Here's how the part is built. I have some questions about the finished solid (model axes, mm). A direction names the side the tool comes from. Give positions to 0.01 mm unless a question says otherwise; leave off trailing zeros. Write each loop counter-clockwise with the first axis right and the second up, starting at its lowest first coordinate (ties: lowest second). Pieces come first, ordered by that corner, then holes. Notation, with made-up numbers: M 25,32.5 L 59,32.5 A14 ccw 59,53.5 Z; hole C -26,56.5 d8. An arc over 180 degrees is marked long. Answer as CSV lines item,"result". Start each with the question number.
Q1. Suppose I cut it at B-B (z = 4). Write out the boundary of the cut face in (x, y), then the cut area to 3 significant figures.
Q2. On a 3-axis mill with a long thin cutter (end or side, diameter ignored), from which of +Z, -Z, +X, -X, +Y, -Y can I reach the whole of each face in a straight line? I mean faces 1 (the cylindrical face through (147.689, 9.598, -62.764)), 2 (the flat face through (148, 2, -87)), 3 (the flat face through (15, 2, -30)). Say none if no direction works.
Q3. Suppose I cut it at C-C (x = 89.25). Write out the boundary of the cut face in (y, z), then the cut area to 3 significant figures.
Q4. Thinking about a two-plate mould opening in X: for faces 4 (the flat face through (36, 2, 0)), 5 (the flat face through (20, 2, -66)), 6 (the flat face through (15, 2, -62)), 7 (the flat face through (37, 2, -67)), which applies, +X half, -X half, draft (parallel to the pull), parting line (faces both ways), or undercut?
Q5. For pin 1 (3.5 mm diameter, centred on x = 27.5, y = 1, fed in from -Z); pin 2 (2 mm diameter, centred on x = 155, y = 1.5, fed in from -Z); pin 3 (1 mm diameter, centred on y = 12, z = -26, fed in from -X), each with a flat end and sliding along its axis, tell me the tip position at first contact or that it passes through.
Q6. Suppose I cut it at A-A (x = 49.5). Write out the boundary of the cut face in (y, z), then the cut area to 4 significant figures.
Q7. If I drill on line 1 along Z through (x, y) = (145.75, 10.25); line 2 along X through (y, z) = (9, 4); line 3 along Z through (x, y) = (145, 1), over which ranges is the centre line in solid material (lowest first)?
```python
from build123d import *
from OCP.BRepFilletAPI import BRepFilletAPI_MakeChamfer

# Parameters (mm, degrees)
SKETCH1_W                       = 180
SKETCH1_H                       = 60
SKETCH1_W_2                     = 150
SKETCH1_H_2                     = 35
BOSS_EXTRUDE1_DEPTH             = 4.5
FILLET1_R                       = 5
FILLET2_R                       = 2
BOSS_EXTRUDE2_DEPTH             = 4.5
CHAMFER1_SIZE                   = 25
CHAMFER2_SIZE                   = 2
BOSS_EXTRUDE3_DEPTH             = 12
BOSS_EXTRUDE3_DIRECTION_2_REACH = 205.581
CHAMFER3_SIZE                   = 10
CHAMFER3_SIZE_2                 = 12
CHAMFER4_SIZE                   = 8
BOSS_EXTRUDE4_START             = 8
BOSS_EXTRUDE4_DEPTH             = 8
SKETCH5_R                       = 2.3
CUT_EXTRUDE1_DEPTH              = 14
CHAMFER5_SIZE                   = 12
CHAMFER5_SIZE2                  = 10
SKETCH6_W                       = 20
SKETCH6_H                       = 10
SKETCH6_W_2                     = 14
SKETCH6_H_2                     = 6
BOSS_EXTRUDE5_DEPTH             = 4.5
CHAMFER6_SIZE                   = 4
SKETCH7_W                       = 14
SKETCH7_H                       = 2.25
CUT_EXTRUDE2_DEPTH              = 3


with BuildPart() as part:
    # Sketch1 → Boss-Extrude1 (new body)
    with BuildSketch(Plane(origin=(0, 0, 0), x_dir=(1, 0, 0), z_dir=(0, 1, 0))):
        with Locations((90, 30)):
            Rectangle(SKETCH1_W, SKETCH1_H)
        with Locations((90, 30)):
            Rectangle(SKETCH1_W_2, SKETCH1_H_2, mode=Mode.SUBTRACT)
    extrude(amount=BOSS_EXTRUDE1_DEPTH)

    # Fillet1
    fillet1_edges = [part.edges().sort_by_distance(p)[0] for p in [
        (0, 2.25, -60),
        (180, 2.25, 0),
        (0, 2.25, 0),
    ]]
    fillet(fillet1_edges, radius=FILLET1_R)

    # Fillet2
    fillet2_edges = [part.edges().sort_by_distance(p)[0] for p in [
        (165, 2.25, -12.5),
        (165, 2.25, -47.5),
        (15, 2.25, -47.5),
        (15, 2.25, -12.5),
    ]]
    fillet(fillet2_edges, radius=FILLET2_R)

    # Sketch2 → Boss-Extrude2 (add)
    with BuildSketch(Plane(origin=(0, 4.5, 0), x_dir=(1, 0, 0), z_dir=(0, 1, 0))):
        Polygon((180, 80), (180, 60), (136, 60), (136, 80), (136, 95), (148, 95), (148, 80), (168, 80), (168, 95), (180, 95), align=None)
    extrude(amount=-BOSS_EXTRUDE2_DEPTH)

    # Chamfer1
    chamfer1_edges = [part.edges().sort_by_distance(p)[0] for p in [
        (136, 2.25, -60),
    ]]
    chamfer(chamfer1_edges, length=CHAMFER1_SIZE)

    # Chamfer2
    chamfer2_edges = [part.edges().sort_by_distance(p)[0] for p in [
        (168, 2.25, -95),
        (148, 2.25, -95),
    ]]
    chamfer(chamfer2_edges, length=CHAMFER2_SIZE)

    # Sketch3 → Boss-Extrude3 (add)
    with BuildSketch(Plane(origin=(0, 4.5, 0), x_dir=(1, 0, 0), z_dir=(0, 1, 0))):
        Polygon((90, -8), (160, -8), (160, 0), (90, 0), (75, 0), (75, -8), align=None)
        Polygon((160, 60), (90, 60), (75, 60), (75, 68), (90, 68), (160, 68), align=None)
    extrude(amount=BOSS_EXTRUDE3_DEPTH)

    # Boss-Extrude3 direction 2: up to this face of the body (flat: up to its plane)
    boss_extrude3_direction_2_end = Plane(part.part.faces().sort_by_distance((141, 0, -92.964686756))[0])
    # Sketch3 → Boss-Extrude3 direction 2 (add, up to the picked face)
    with BuildSketch(Plane(origin=(0, 4.5, 0), x_dir=(1, 0, 0), z_dir=(0, 1, 0)), mode=Mode.PRIVATE) as boss_extrude3_direction_2_sk1:
        Polygon((90, -8), (160, -8), (160, 0), (90, 0), (75, 0), (75, -8), align=None)
    boss_extrude3_direction_2_tool1 = split(extrude(boss_extrude3_direction_2_sk1.sketch, amount=-BOSS_EXTRUDE3_DIRECTION_2_REACH, mode=Mode.PRIVATE), bisect_by=boss_extrude3_direction_2_end, keep=Keep.BOTH, mode=Mode.PRIVATE)
    # Sketch3 → Boss-Extrude3 direction 2 (add, up to the picked face)
    with BuildSketch(Plane(origin=(0, 4.5, 0), x_dir=(1, 0, 0), z_dir=(0, 1, 0)), mode=Mode.PRIVATE) as boss_extrude3_direction_2_sk2:
        Polygon((160, 60), (90, 60), (75, 60), (75, 68), (90, 68), (160, 68), align=None)
    boss_extrude3_direction_2_tool2 = split(extrude(boss_extrude3_direction_2_sk2.sketch, amount=-BOSS_EXTRUDE3_DIRECTION_2_REACH, mode=Mode.PRIVATE), bisect_by=boss_extrude3_direction_2_end, keep=Keep.BOTH, mode=Mode.PRIVATE)
    add(boss_extrude3_direction_2_tool1.solids().sort_by(Axis((117.5, 4.5, 4), (0, -1, 0)))[0])
    add(boss_extrude3_direction_2_tool2.solids().sort_by(Axis((117.5, 4.5, -64), (0, -1, 0)))[0])

    # Chamfer3
    chamfer3_edges_1 = [part.edges().sort_by_distance(p)[0] for p in [
        (160, 16.5, -64),
    ]]
    chamfer3_side_1 = [part.faces().sort_by_distance(p)[0] for p in [
        (159.8, 16.5, -64),
    ]]
    chamfer3_edges_2 = [part.edges().sort_by_distance(p)[0] for p in [
        (75, 16.5, -64),
    ]]
    chamfer3_side_2 = [part.faces().sort_by_distance(p)[0] for p in [
        (75.2, 16.5, -64),
    ]]
    chamfer3_edges_3 = [part.edges().sort_by_distance(p)[0] for p in [
        (75, 16.5, 4),
    ]]
    chamfer3_side_3 = [part.faces().sort_by_distance(p)[0] for p in [
        (75.2, 16.5, 4),
    ]]
    chamfer3 = BRepFilletAPI_MakeChamfer(part.part.solid().wrapped)
    for e in chamfer3_edges_1:
        chamfer3.Add(CHAMFER3_SIZE - 0.0001, CHAMFER3_SIZE_2 - 0.0001, e.wrapped, chamfer3_side_1[0].wrapped)
    for e in chamfer3_edges_2:
        chamfer3.Add(CHAMFER3_SIZE - 0.0001, CHAMFER3_SIZE_2 - 0.0001, e.wrapped, chamfer3_side_2[0].wrapped)
    for e in chamfer3_edges_3:
        chamfer3.Add(CHAMFER3_SIZE - 0.0001, CHAMFER3_SIZE_2 - 0.0001, e.wrapped, chamfer3_side_3[0].wrapped)
    add(Compound.cast(chamfer3.Shape()), mode=Mode.REPLACE)  # a hair under: the kernel refuses the full size

    # Chamfer4
    chamfer4_edges = [part.edges().sort_by_distance(p)[0] for p in [
        (160, 2.25, 0),
        (75, 2.25, 0),
        (75, 2.25, -60),
    ]]
    chamfer(chamfer4_edges, length=CHAMFER4_SIZE - 0.0001)  # a hair under: the kernel refuses the full size

    # Sketch4 → Boss-Extrude4 (add)
    with BuildSketch(Plane(origin=(0, 4.5, 0), x_dir=(1, 0, 0), z_dir=(0, 1, 0)).offset(BOSS_EXTRUDE4_START)):
        with BuildLine():
            Line((180, 95), (180, 5))
            ThreePointArc((180, 5), (178.535533906, 1.464466094), (175, 0))
            Line((175, 0), (172, 0))
            Line((172, 0), (172, 95))
            Line((172, 95), (180, 95))
        make_face()
    extrude(amount=-BOSS_EXTRUDE4_DEPTH)

    # Sketch5 → Cut-Extrude1 (cut)
    with BuildSketch(Plane(origin=(0, 16.5, 0), x_dir=(1, 0, 0), z_dir=(0, 1, 0))):
        with Locations(Location((89.25, 64, 0), (0, 0, 270))):
            Circle(SKETCH5_R)
        with Locations(Location((145.75, 64, 0), (0, 0, 270))):
            Circle(SKETCH5_R)
        with Locations(Location((145.75, -4, 0), (0, 0, 270))):
            Circle(SKETCH5_R)
        with Locations(Location((89.25, -4, 0), (0, 0, 270))):
            Circle(SKETCH5_R)
    extrude(amount=-CUT_EXTRUDE1_DEPTH, mode=Mode.SUBTRACT)

    # Chamfer5
    chamfer5_edges = [part.edges().sort_by_distance(p)[0] for p in [
        (160, 16.5, 4),
    ]]
    chamfer5_side = [part.faces().sort_by_distance(p)[0] for p in [
        (160, 10.499961328, 4.00001875),
    ]]
    chamfer(chamfer5_edges, length=CHAMFER5_SIZE, length2=CHAMFER5_SIZE2, reference=chamfer5_side[0])

    # Sketch6 → Boss-Extrude5 (add)
    # profile 1 of 2: a face of its own
    with BuildSketch(Plane(origin=(0, 4.5, 0), x_dir=(1, 0, 0), z_dir=(0, 1, 0))):
        with Locations((27, 65)):
            Rectangle(SKETCH6_W, SKETCH6_H)
        with Locations((27, 65)):
            Rectangle(SKETCH6_W_2, SKETCH6_H_2, mode=Mode.SUBTRACT)
    # profile 2 of 2: a face of its own
    with BuildSketch(Plane(origin=(0, 4.5, 0), x_dir=(1, 0, 0), z_dir=(0, 1, 0))):
        with BuildLine():
            Line((168, 0), (172, 0))
            Line((172, 0), (172, 95))
            Line((172, 95), (170, 95))
            Line((170, 95), (168, 93))
            Line((168, 93), (168, 80))
            Line((168, 80), (148, 80))
            Line((148, 80), (148, 93))
            Line((148, 93), (146, 95))
            Line((146, 95), (136, 95))
            Line((136, 95), (136, 85))
            Line((136, 85), (119, 68))
            Line((119, 68), (160, 68))
            Line((160, 68), (160, 60))
            Line((160, 60), (75, 60))
            Line((75, 60), (75, 68))
            Line((75, 68), (67, 60))
            Line((67, 60), (5, 60))
            ThreePointArc((5, 60), (1.464466094, 58.535533906), (0, 55))
            Line((0, 55), (0, 5))
            ThreePointArc((0, 5), (1.464466094, 1.464466094), (5, 0))
            Line((5, 0), (67, 0))
            Line((67, 0), (75, -8))
            Line((75, -8), (75, 0))
            Line((75, 0), (160, 0))
            Line((160, 0), (160, -8))
            Line((160, -8), (168, 0))
        make_face()
        with BuildLine():
            ThreePointArc((163, 47.5), (164.414213562, 46.914213562), (165, 45.5))
            Line((165, 45.5), (165, 14.5))
            ThreePointArc((165, 14.5), (164.414213562, 13.085786438), (163, 12.5))
            Line((163, 12.5), (17, 12.5))
            ThreePointArc((17, 12.5), (15.585786438, 13.085786438), (15, 14.5))
            Line((15, 14.5), (15, 45.5))
            ThreePointArc((15, 45.5), (15.585786438, 46.914213562), (17, 47.5))
            Line((17, 47.5), (163, 47.5))
        make_face(mode=Mode.SUBTRACT)
    extrude(amount=-BOSS_EXTRUDE5_DEPTH)

    # Chamfer6
    chamfer6_edges = [part.edges().sort_by_distance(p)[0] for p in [
        (17, 2.25, -60),
        (37, 2.25, -60),
    ]]
    chamfer(chamfer6_edges, length=CHAMFER6_SIZE)

    # Sketch7 → Cut-Extrude2 (cut)
    with BuildSketch(Plane.XY.offset(-68)):
        with Locations((27, 1.125)):
            Rectangle(SKETCH7_W, SKETCH7_H)
    extrude(amount=-CUT_EXTRUDE2_DEPTH, mode=Mode.SUBTRACT)


solid = part.part
```
Resolved:
1,outline,"M 71,0 L 164,0 L 164,4.5 L 160,4.5 L 150,16.5 L 148.05,16.5 L 148.05,2.5 L 143.45,2.5 L 143.45,16.5 L 91.55,16.5 L 91.55,2.5 L 86.95,2.5 L 86.95,16.5 L 85,16.5 L 75,4.5 L 71,4.5 Z"
1,area,"1,190 mm^2"
2,face 1,"+Y"
2,face 2,"-Z, +Y, -Y"
2,face 3,"+Y, -Y"
3,outline,"M 0,-68 L 16.5,-68 L 16.5,-66.3 L 2.5,-66.3 L 2.5,-61.7 L 16.5,-61.7 L 16.5,-60 L 4.5,-60 L 4.5,-47.5 L 0,-47.5 Z; M 0,-12.5 L 4.5,-12.5 L 4.5,0 L 16.5,0 L 16.5,1.7 L 2.5,1.7 L 2.5,6.3 L 16.5,6.3 L 16.5,8 L 0,8 Z"
3,area,"248 mm^2"
4,face 4,"draft"
4,face 5,"undercut"
4,face 6,"-X half"
4,face 7,"undercut"
5,pin 1,"z = -70"
5,pin 2,"z = -80"
5,pin 3,"x = 172"
6,outline,"M 0,-60 L 4.5,-60 L 4.5,-47.5 L 0,-47.5 Z; M 0,-12.5 L 4.5,-12.5 L 4.5,0 L 0,0 Z"
6,area,"112.5 mm^2"
7,line 1,"-68 to -66.3, -61.7 to -60, 0 to 1.7, 6.3 to 8"
7,line 2,"78.75 to 86.95, 91.55 to 143.45, 148.05 to 156.25"
7,line 3,"-95 to -47.5, -12.5 to 8"
